Verification items for the finished model (mm, model axes). Face numbers are marked on the shaded views. A direction names the side the tool comes from. Give positions to 0.01 mm unless a question says otherwise; leave off trailing zeros. Loops run counter-clockwise (first coordinate to the right, second up) from the corner with the lowest first, then second, coordinate; pieces in that order, holes last. Notation, with made-up numbers: (-33.75, 24.25) -> (-28.75, 24.25) arc R25 cw to (-28.75, 63.25) -> close; hole circle Ø7 at (19, -16). An arc over 180 degrees is marked (long way). Answer in a Markdown table with one row per item. Add a question column.
Q1. Gauge pin test, flat ends, axial feed: P1, Ø2, axis at x = 9, z = -0.5, coming from the +Y side; P2, Ø2, axis at x = -5.5, z = 0.5, coming from the -Y side; P3, Ø1, axis at x = 9, z = -1.5, coming from the -Y side. Record the tip position at first contact, or that the pin passes through.
Q2. Section check B-B on z = -1.05. Enter the section's corners in (x, y) (3 decimals), and give its area (3 significant figures).
Q3. Set-up check for the marked faces 1, 2 and 3: record each of +Z, -Z, +X, -X, +Y, -Y from which the full face is reachable in a straight line by a thin tool's end or side.
Q4. Section check A-A on x = -3.5. Enter the section's corners in (y, z).
Q5. Section check C-C on x = 6. Enter the section's corners in (y, z), and give its area (3 significant figures).
Q6. Material ranges on probe 1 along Y at (x, z) = (5, -0.45); probe 2 along Z at (x, y) = (-8, -0.5); probe 3 along Z at (x, y) = (0, -3.5), recorded low to high.
```python
from build123d import *

# Parameters (mm, degrees)
F1_DEPTH    = 2
F2_T1_DEPTH = 25.25
F2_T4_ANGLE = 180
F2_T6_ANGLE = 180
F4_DEPTH    = 2


# Not quite as in the source:
# - a fillet or chamfer that OpenCascade refuses, or shapes differently, is made with other operations: its cross-section is extruded or revolved along the edge and cut away or added


with BuildPart() as f1:
    # F0 (on Top) → F1 (new body)
    with BuildSketch(Plane.XY):
        with BuildLine():
            Line((-12.625, -7.5), (12.625, -7.5))
            ThreePointArc((12.625, -7.5), (20.125, 0), (12.625, 7.5))
            Line((12.625, 7.5), (-12.625, 7.5))
            ThreePointArc((-12.625, 7.5), (-20.125, 0), (-12.625, -7.5))
        make_face()
    extrude(amount=F1_DEPTH)

    # F2: fillet of radius 14 on 1 edges, made by hand

    # F2_s2 → F2_t1 (cut)
    with BuildSketch(Plane.YZ.offset(-12.625)):
        with BuildLine():
            ThreePointArc((7.5, 0), (4.0305548358, 1.4907375632), (0.2888974491, 2))
            Line((0.2888974491, 2), (0.2888974491, 2.28))
            Line((0.2888974491, 2.28), (7.5, 2.28))
            Line((7.5, 2.28), (7.78, 2))
            ThreePointArc((7.78, 2), (7.78, 1), (7.644222051, 0.24))
            Line((7.644222051, 0.24), (7.5, 0))
        make_face()
        with BuildLine():
            ThreePointArc((-7.5, 0), (-4.0305548358, 1.4907375632), (-0.2888974491, 2))
            Line((-0.2888974491, 2), (-0.2888974491, 2.28))
            Line((-0.2888974491, 2.28), (-7.5, 2.28))
            Line((-7.5, 2.28), (-7.78, 2))
            ThreePointArc((-7.78, 2), (-7.78, 1), (-7.644222051, 0.24))
            Line((-7.644222051, 0.24), (-7.5, 0))
        make_face()
    extrude(amount=F2_T1_DEPTH, mode=Mode.SUBTRACT)

    # F2_s3 → F2_t4 (revolve, cut)
    with BuildSketch(Plane.YZ.offset(12.625)):
        with BuildLine():
            ThreePointArc((-7.5, 0), (-4.0305548358, 1.4907375632), (-0.2888974491, 2))
            Line((-0.2888974491, 2), (-0.2888974491, 2.28))
            Line((-0.2888974491, 2.28), (-7.5, 2.28))
            Line((-7.5, 2.28), (-7.78, 2))
            ThreePointArc((-7.78, 2), (-7.78, 1), (-7.644222051, 0.24))
            Line((-7.644222051, 0.24), (-7.5, 0))
        make_face()
    revolve(axis=Axis((12.625, 0, 2), (0, 0, 1)), revolution_arc=F2_T4_ANGLE, mode=Mode.SUBTRACT)

    # F2_s5 → F2_t6 (revolve, cut)
    with BuildSketch(Plane.YZ.offset(-12.625)):
        with BuildLine():
            ThreePointArc((7.5, 0), (4.0305548358, 1.4907375632), (0.2888974491, 2))
            Line((0.2888974491, 2), (0.2888974491, 2.28))
            Line((0.2888974491, 2.28), (7.5, 2.28))
            Line((7.5, 2.28), (7.78, 2))
            ThreePointArc((7.78, 2), (7.78, 1), (7.644222051, 0.24))
            Line((7.644222051, 0.24), (7.5, 0))
        make_face()
    revolve(axis=Axis((-12.625, 0, 2), (0, 0, 1)), revolution_arc=F2_T6_ANGLE, mode=Mode.SUBTRACT)

    # F3 (on face) → F4 (join)
    with BuildSketch(Plane(origin=(0, 0, 0), x_dir=(1, 0, 0), z_dir=(0, 0, -1))):
        with BuildLine():
            ThreePointArc((18.1022727273, 0.499483204), (16.3332908717, 4.0618442623), (12.625, 5.5))
            Line((12.625, 5.5), (6.5, 5.5))
            ThreePointArc((6.5, 5.5), (6, 6), (5.5, 5.5))
            Line((5.5, 5.5), (-5.5, 5.5))
            ThreePointArc((-5.5, 5.5), (-6, 6), (-6.5, 5.5))
            Line((-6.5, 5.5), (-12.625, 5.5))
            ThreePointArc((-12.625, 5.5), (-16.3332908717, 4.0618442623), (-18.1022727273, 0.499483204))
            ThreePointArc((-18.1022727273, 0.499483204), (-18.625, 0), (-18.1022727273, -0.499483204))
            ThreePointArc((-18.1022727273, -0.499483204), (-16.3332908717, -4.0618442623), (-12.625, -5.5))
            Line((-12.625, -5.5), (-6.5, -5.5))
            ThreePointArc((-6.5, -5.5), (-6, -6), (-5.5, -5.5))
            Line((-5.5, -5.5), (5.5, -5.5))
            ThreePointArc((5.5, -5.5), (6, -6), (6.5, -5.5))
            Line((6.5, -5.5), (12.625, -5.5))
            ThreePointArc((12.625, -5.5), (16.3332908717, -4.0618442623), (18.1022727273, -0.499483204))
            ThreePointArc((18.1022727273, -0.499483204), (18.625, 0), (18.1022727273, 0.499483204))
        make_face()
    extrude(amount=F4_DEPTH)


solid = f1.part
```
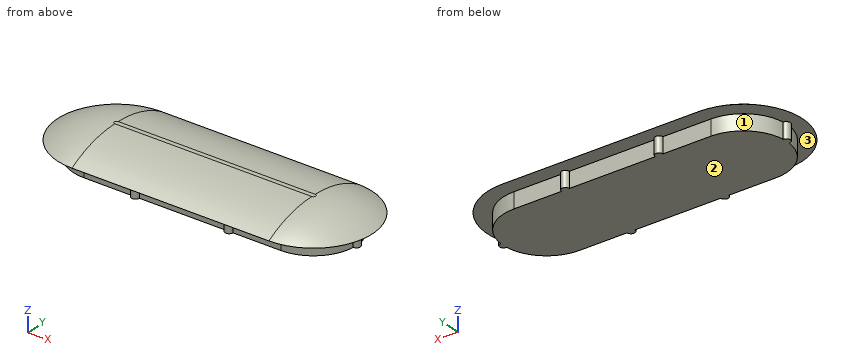
Taken from the geometry:
| question | item | result |
|---|---|---|
| 1 | P1 | stops at y = 7.5 |
| 1 | P2 | stops at y = -7.5 |
| 1 | P3 | stops at y = -5.5 |
| 2 | outline | (-18.102, -0.499) arc R5.5 ccw to (-12.625, -5.5) -> (-6.5, -5.5) arc R0.5 ccw to (-5.5, -5.5) -> (5.5, -5.5) arc R0.5 ccw to (6.5, -5.5) -> (12.625, -5.5) arc R5.5 ccw to (18.102, -0.499) arc R0.5 ccw (long way) to (18.102, 0.499) arc R5.5 ccw to (12.625, 5.5) -> (6.5, 5.5) arc R0.5 ccw to (5.5, 5.5) -> (-5.5, 5.5) arc R0.5 ccw to (-6.5, 5.5) -> (-12.625, 5.5) arc R5.5 ccw to (-18.102, 0.499) arc R0.5 ccw (long way) to start |
| 2 | area | 375 mm² |
| 3 | face 1 | -Z, -X, +Y |
| 3 | face 2 | -Z, +X, -X, +Y, -Y |
| 3 | face 3 | -Z |
| 4 | outline | (-7.5, 0) -> (-5.5, 0) -> (-5.5, -2) -> (5.5, -2) -> (5.5, 0) -> (7.5, 0) arc R14 ccw to (0.29, 2) -> (-0.29, 2) arc R14 ccw to start |
| 5 | outline | (-7.5, 0) -> (-6, 0) -> (-6, -2) -> (6, -2) -> (6, 0) -> (7.5, 0) arc R14 ccw to (0.29, 2) -> (-0.29, 2) arc R14 ccw to start |
| 5 | area | 44.7 mm² |
| 6 | probe 1 | y = -5.5 to 5.5 |
| 6 | probe 2 | z = -2 to 2 |
| 6 | probe 3 | z = -2 to 1.63 |
